from build123d import *

# Parameters (mm, degrees)
SKETCH1_R           = 3.149606299
BOSS_EXTRUDE1_DEPTH = 28.575
CUT_EXTRUDE1_DEPTH  = 19.304
CUT_EXTRUDE7_DEPTH  = 6.35
SKETCH5_R           = 4
CUT_EXTRUDE3_DEPTH  = 31


with BuildPart() as part:
    # Sketch1 → Boss-Extrude1 (new body)
    with BuildSketch(Plane(origin=(0, 0, 0), x_dir=(1, 0, 0), z_dir=(0, 1, 0))):
        Polygon((0, 6.666666667), (0, 23.333333333), (0, 30), (6.666666667, 30), (93.333333333, 30), (100, 30), (100, 0), (93.333333333, 0), (6.666666667, 0), (0, 0), align=None)
        with Locations((13.333333333, 15)):
            Circle(SKETCH1_R, mode=Mode.SUBTRACT)
        with Locations((53.333333333, 15)):
            Circle(SKETCH1_R, mode=Mode.SUBTRACT)
    extrude(amount=-BOSS_EXTRUDE1_DEPTH)

    # Sketch2 → Cut-Extrude1 (cut)
    with BuildSketch(Plane(origin=(0, 0, 0), x_dir=(1, 0, 0), z_dir=(0, 1, 0))):
        with BuildLine():
            Line((3.810000003, 6.985), (3.810000003, 21.59))
            ThreePointArc((3.810000003, 21.59), (4.739935973, 23.83506403), (6.985000003, 24.765))
            Line((6.985000003, 24.765), (59.678333333, 24.765))
            ThreePointArc((59.678333333, 24.765), (61.923397364, 23.83506403), (62.853333333, 21.59))
            Line((62.853333333, 21.59), (62.853333333, 6.985))
            ThreePointArc((62.853333333, 6.985), (61.923397364, 4.73993597), (59.678333333, 3.81))
            Line((59.678333333, 3.81), (6.985000003, 3.81))
            ThreePointArc((6.985000003, 3.81), (4.739935973, 4.73993597), (3.810000003, 6.985))
        make_face()
        with BuildLine():
            Line((66.853333333, 6.985), (66.853333333, 21.59))
            ThreePointArc((66.853333333, 21.59), (67.783269303, 23.83506403), (70.028333333, 24.765))
            Line((70.028333333, 24.765), (95.25, 24.765))
            Line((95.25, 24.765), (95.25, 3.81))
            Line((95.25, 3.81), (70.028333333, 3.81))
            ThreePointArc((70.028333333, 3.81), (67.783269303, 4.73993597), (66.853333333, 6.985))
        make_face()
    extrude(amount=-CUT_EXTRUDE1_DEPTH, mode=Mode.SUBTRACT)

    # Sketch9 → Cut-Extrude7 (cut)
    with BuildSketch(Plane(origin=(0, -19.304, 0), x_dir=(1, 0, 0), z_dir=(0, 1, 0))):
        with BuildLine():
            Line((7.649092718, 18.135984848), (10.793997252, 22.263484848))
            ThreePointArc((10.793997252, 22.263484848), (13.026694001, 24.105359338), (15.844904534, 24.765))
            Line((15.844904534, 24.765), (50.818428803, 24.765))
            ThreePointArc((50.818428803, 24.765), (53.636639335, 24.105359338), (55.869336085, 22.263484848))
            Line((55.869336085, 22.263484848), (59.014240619, 18.135984848))
            ThreePointArc((59.014240619, 18.135984848), (60.313333337, 14.2875), (59.014240619, 10.439015152))
            Line((59.014240619, 10.439015152), (55.869336085, 6.311515152))
            ThreePointArc((55.869336085, 6.311515152), (53.636639335, 4.469640662), (50.818428803, 3.81))
            Line((50.818428803, 3.81), (15.844904534, 3.81))
            ThreePointArc((15.844904534, 3.81), (13.026694001, 4.469640662), (10.793997252, 6.311515152))
            Line((10.793997252, 6.311515152), (7.649092718, 10.439015152))
            ThreePointArc((7.649092718, 10.439015152), (6.35, 14.2875), (7.649092718, 18.135984848))
        make_face()
        with BuildLine():
            Line((66.853333333, 18.415), (66.853333333, 10.16))
            ThreePointArc((66.853333333, 10.16), (68.713205273, 5.669871939), (73.203333333, 3.81))
            Line((73.203333333, 3.81), (95.25, 3.81))
            Line((95.25, 3.81), (95.25, 24.765))
            Line((95.25, 24.765), (73.203333333, 24.765))
            ThreePointArc((73.203333333, 24.765), (68.713205273, 22.905128061), (66.853333333, 18.415))
        make_face()
    extrude(amount=-CUT_EXTRUDE7_DEPTH, mode=Mode.SUBTRACT)

    # Sketch5 → Cut-Extrude3 (cut, through all)
    with BuildSketch(Plane(origin=(0, 0, -30), x_dir=(-1, 0, 0), z_dir=(0, 0, -1))):
        with BuildLine():
            Line((0, 0), (-31.75, 0))
            ThreePointArc((-31.75, 0), (-29.462234044, -0.278825011), (-27.308407483, -1.098975973))
            Line((-27.308407483, -1.098975973), (-3.388938322, -13.707595992))
            ThreePointArc((-3.388938322, -13.707595992), (-0.912848096, -16.044719868), (0, -19.324945344))
            Line((0, -19.324945344), (0, 0))
        make_face()
        with BuildLine():
            ThreePointArc((0, -22.225), (-1.859871939, -26.715128061), (-6.35, -28.575))
            Line((-6.35, -28.575), (0, -28.575))
            Line((0, -28.575), (0, -22.225))
        make_face()
        with BuildLine():
            Line((-77.893333333, -27.305), (-91.44, -17.145))
            ThreePointArc((-91.44, -17.145), (-94.761208414, -6.512930529), (-85.725, 0))
            Line((-85.725, 0), (-100, 0))
            Line((-100, 0), (-100, -28.575))
            Line((-100, -28.575), (-74.083333333, -28.575))
            ThreePointArc((-74.083333333, -28.575), (-76.091379648, -28.249138943), (-77.893333333, -27.305))
        make_face()
        with Locations((-85.725, -9.525)):
            Circle(SKETCH5_R)
        with Locations((-31.75, -9.525)):
            Circle(SKETCH5_R)
    extrude(amount=-CUT_EXTRUDE3_DEPTH, mode=Mode.SUBTRACT)


solid = part.part
Build history of the part. All positions in model axes, mm. A direction names the side the tool comes from. Round coordinates to 2 decimals unless told otherwise and drop trailing zeros. Loops run counter-clockwise (first coordinate to the right, second up) from the corner with the lowest first, then second, coordinate; pieces in that order, holes last. Notation, with made-up numbers: (47.25, 61) -> (106.25, 61) arc R8 ccw to (106.25, 72) -> close; hole circle Ø1 at (-24.5, -40). An arc over 180 degrees is marked (long way). One line per item, written item: value. Start each with the question number.
Q1. Cut at C-C on y = -15.75. List the corners of the cut face in (x, z) (3 decimals), plus the area to 3 significant figures.
Q2. Cut at D-D on y = -8.5. Count the separate pieces of the cut face and the enclosed holes in it, plus the area to 3 significant figures.
Q3. Drop flat-ended pins along their axis: pin 1 Ø1.9 at (x, z) = (70.5, -7) entering from +Y; pin 2 Ø13 at (x, z) = (55.5, -19) entering from +Y; pin 3 Ø1.9 at (x, z) = (69, -23) entering from +Y; pin 4 Ø1.5 at (y, z) = (-6, -15) entering from +X. Give the stop position or say it passes through.
Q4. Two-plate mould, pull along Y, no slides. Class faces 1 (the face through (34.924, -11.959, -27.419)), 2 (the face through (4.76, -16.34, -4.72)), 3 (the face through (15.404, -7.374, -25.07)): released by +Y, released by -Y, zero draft, split by the parting line, or undercut.
Q5. Cut at B-B on x = 38.5. List the corners of the cut face in (y, z) (3 decimals).
Q6. 3-axis set-ups, long thin cutter, end or side, ignore diameter. For faces 4 (the face through (65, 0, -19)), 5 (the face through (67.808, -9.517, -4.715)), 6 (the face through (12.99, -22.435, -24.087)): which of +Z, -Z, +X, -X, +Y, -Y reach the whole face in a straight line?
Q7. Cut at A-A on z = -15. List the corners of the cut face in (x, y) (3 decimals).
Q8. Probe line 1 along Z through (x, y) = (37.5, -3.25) (3 decimals); line 2 along X through (y, z) = (-26.6, -15); line 3 along X through (y, z) = (-26.5, -15). List the from-to ranges inside material, lowest first.
Computed:
1. outline: (1.102, -30) -> (92.934, -30) -> (92.934, -24.765) -> (70.028, -24.765) arc R3.175 cw to (66.853, -21.59) -> (66.853, -6.985) arc R3.175 cw to (70.028, -3.81) -> (92.934, -3.81) -> (92.934, 0) -> (1.102, 0) -> close; hole (3.81, -21.59) arc R3.175 ccw to (6.985, -24.765) -> (59.678, -24.765) arc R3.175 ccw to (62.853, -21.59) -> (62.853, -6.985) arc R3.175 ccw to (59.678, -3.81) -> (6.985, -3.81) arc R3.175 ccw to (3.81, -6.985) -> close
1. area: 984 mm²
2. separate pieces: 5
2. enclosed holes: 0
2. area: 694 mm²
3. pin 1: y = -25.65
3. pin 2: y = 0
3. pin 3: y = -19.3
3. pin 4: x = 66.85
4. face 1: undercut
4. face 2: zero draft
4. face 3: released by +Y
5. outline: (-28.575, -30) -> (0, -30) -> (0, -24.765) -> (-25.654, -24.765) -> (-25.654, -3.81) -> (0, -3.81) -> (0, 0) -> (-28.575, 0) -> close
6. face 4: +Z, -Z, +X, -X, +Y
6. face 5: +X, +Y
6. face 6: +Y
7. outline: (0, -22.225) arc R6.35 ccw to (6.35, -28.575) -> (10.184, -28.575) -> (10.184, -25.654) -> (6.39, -25.654) -> (6.39, -19.304) -> (3.81, -19.304) -> (3.81, -13.486) -> (3.389, -13.708) arc R6.35 ccw to (0, -19.325) -> close; (16.483, -28.575) -> (50.184, -28.575) -> (50.184, -25.654) -> (16.483, -25.654) -> close; (56.483, -28.575) -> (74.083, -28.575) arc R6.35 ccw to (77.893, -27.305) -> (80.095, -25.654) -> (66.853, -25.654) -> (66.853, 0) -> (62.853, 0) -> (62.853, -19.304) -> (60.273, -19.304) -> (60.273, -25.654) -> (56.483, -25.654) -> close
8. line 1: -30 to -24.765, -3.81 to 0
8. line 2: 1.75 to 10.18, 16.48 to 50.18, 56.48 to 78.83
8. line 3: 1.65 to 10.18, 16.48 to 50.18, 56.48 to 78.97
